```python
from build123d import *

# Parameters (mm, degrees)
BOSS_EXTRUDE1_DEPTH = 0.8
SKETCH3_W           = 6.4
SKETCH3_H           = 0.5
BOSS_EXTRUDE2_DEPTH = 0.2
BOSS_EXTRUDE3_DEPTH = 0.4
SKETCH5_R           = 1.1
BOSS_EXTRUDE4_DEPTH = 0.4
FILLET2_R           = 0.1
FILLET3_R           = 0.1
FILLET4_R           = 0.1


with BuildPart() as part:
    # Sketch1 → Boss-Extrude1 (new body)
    with BuildSketch(Plane.XY):
        Polygon((-1.3, 2.6), (1.3, 2.6), (1.3, 2.2), (2.2, 1.3), (2.6, 1.3), (2.6, -1.3), (2.2, -1.3), (1.3, -2.2), (1.3, -2.6), (-1.3, -2.6), (-1.3, -2.2), (-2.2, -1.3), (-2.6, -1.3), (-2.6, 1.3), (-2.2, 1.3), (-1.3, 2.2), align=None)
    extrude(amount=BOSS_EXTRUDE1_DEPTH)

    # Sketch3 → Boss-Extrude2 (add)
    with BuildSketch(Plane.XY):
        with Locations((0, 1.95)):
            Rectangle(SKETCH3_W, SKETCH3_H)
        with Locations((0, -1.95)):
            Rectangle(SKETCH3_W, SKETCH3_H)
    extrude(amount=BOSS_EXTRUDE2_DEPTH)

    # Sketch4 → Boss-Extrude3 (add)
    with BuildSketch(Plane.XY.offset(0.8)):
        Polygon((-0.875, 1.75), (0.875, 1.75), (1.75, 0.875), (1.75, -0.875), (0.875, -1.75), (-0.875, -1.75), (-1.75, -0.875), (-1.75, 0.875), align=None)
    extrude(amount=BOSS_EXTRUDE3_DEPTH)

    # Sketch5 → Boss-Extrude4 (add)
    with BuildSketch(Plane.XY.offset(1.2)):
        with Locations(Location((0, 0, 0), (0, 0, 180))):
            Circle(SKETCH5_R)
    extrude(amount=BOSS_EXTRUDE4_DEPTH)

    # Fillet2
    fillet2_edges = [part.edges().sort_by_distance(p)[0] for p in [
        (1.1, 0, 1.6),
    ]]
    fillet(fillet2_edges, radius=FILLET2_R)

    # Fillet3
    fillet3_edges = [part.edges().sort_by_distance(p)[0] for p in [
        (1.3, 2.4, 0.8),
        (0, 2.6, 0.8),
        (-1.3, 2.4, 0.8),
        (-1.75, 1.75, 0.8),
        (-2.4, 1.3, 0.8),
        (-2.6, 0, 0.8),
        (-2.4, -1.3, 0.8),
        (-1.75, -1.75, 0.8),
        (-1.3, -2.4, 0.8),
        (0, -2.6, 0.8),
        (2.4, 1.3, 0.8),
        (1.3, -2.4, 0.8),
        (1.75, -1.75, 0.8),
        (2.4, -1.3, 0.8),
        (2.6, 0, 0.8),
        (1.75, 1.75, 0.8),
        (1.3125, 1.3125, 0.8),
        (0, 1.75, 0.8),
        (-1.3125, 1.3125, 0.8),
        (-1.75, 0, 0.8),
        (-1.3125, -1.3125, 0.8),
        (0, -1.75, 0.8),
        (1.3125, -1.3125, 0.8),
        (1.75, 0, 0.8),
    ]]
    fillet(fillet3_edges, radius=FILLET3_R)

    # Fillet4
    fillet4_edges = [part.edges().sort_by_distance(p)[0] for p in [
        (0, 1.75, 1.2),
        (-1.3125, 1.3125, 1.2),
        (-1.75, 0, 1.2),
        (-1.3125, -1.3125, 1.2),
        (0, -1.75, 1.2),
        (1.3125, -1.3125, 1.2),
        (1.75, 0, 1.2),
        (1.3125, 1.3125, 1.2),
    ]]
    fillet(fillet4_edges, radius=FILLET4_R)


solid = part.part
```
Geometry: final body of the model. Coordinates: model frame, mm. A direction names the side the tool comes from. Coordinates: 2 decimals unless noted, no trailing zeros. Order: outer loops, then holes, each group sorted by start corner. A loop starts at its lowest first (then second) coordinate and runs counter-clockwise, first axis right, second up. Notation, with made-up numbers: (51.5, 53) -> (66.5, 53) arc R15 ccw to (66.5, 58) -> close; hole circle Ø3 at (-8, -20). An arc over 180 degrees is marked (long way). Write each question's results on one line, items separated by ' | '. Start each with the question number.
1) Cut plane A-A, the plane x = 0. Output: boundary loops of the cut face in (y, z), and give its area (3 significant figures).
2) First-contact query: pin 1 (0.6 mm diameter, centred on y = 0.5, z = 0.5, fed in from +X). Flat tip, straight axial feed; report the tip coordinate or a pass-through.
3) Set-up query: faces 1 (the flat face through (2, 1, 0.8)), 2 (the flat face through (0, 0, 1.6)). Return all of +Z, -Z, +X, -X, +Y, -Y with unobstructed straight access to the full face (end or side cutting, diameter ignored); none if empty.
4) Material intervals for line 1 along Z through (x, y) = (0.75, 1.1); line 2 along X through (y, z) = (0.7, 0.6); line 3 along Z through (x, y) = (-2.25, -0.9), sorted ascending.
5) Cut plane C-C, the plane x = 2. State how many separate pieces and enclosed holes the cut face has, and give its area (3 significant figures).
Checks:
1) outline: (-2.6, 0) -> (2.6, 0) -> (2.6, 0.7) arc R0.1 ccw to (2.5, 0.8) -> (1.85, 0.8) arc R0.1 cw to (1.75, 0.9) -> (1.75, 1.1) arc R0.1 ccw to (1.65, 1.2) -> (1.1, 1.2) -> (1.1, 1.5) arc R0.1 ccw to (1, 1.6) -> (-1, 1.6) arc R0.1 ccw to (-1.1, 1.5) -> (-1.1, 1.2) -> (-1.65, 1.2) arc R0.1 ccw to (-1.75, 1.1) -> (-1.75, 0.9) arc R0.1 cw to (-1.85, 0.8) -> (-2.5, 0.8) arc R0.1 ccw to (-2.6, 0.7) -> close | area: 6.43 mm^2
2) pin 1: x = 2.6
3) face 1: +Z | face 2: +Z, +X, -X, +Y, -Y
4) line 1: 0 to 1.2 | line 2: -2.6 to 2.6 | line 3: 0 to 0.8
5) separate pieces: 3 | enclosed holes: 0 | area: 2.59 mm^2
